from build123d import *

# Parameters (mm, degrees)
F0_R           = 25.1
F1_DEPTH       = 30
F2_R           = 2
F5_D           = 20
F5_DEPTH       = 190
F5_CSINK_D     = 22
F5_CSINK_ANGLE = 90
F5_TIP         = 6.0086061903


# Not quite as in the source:
# - a feature of the source that left no trace in its solid (it failed there, or was rolled back) is left out


with BuildPart() as f1:
    # F0 (on Front) → F1 (new body)
    with BuildSketch(Plane.XZ):
        with Locations((20.5169470484, 0)):
            Circle(F0_R)
    extrude(amount=F1_DEPTH)

    # F2
    f2_edges = [f1.edges().sort_by_distance(p)[0] for p in [
        (-4.583053, 0, 0),
    ]]
    fillet(f2_edges, radius=F2_R)

    # F5
    with Locations(Plane(origin=(0, 0, 0), x_dir=(-1, 0, 0), z_dir=(0, 1, 0))):
        with Locations((-20.5169470484, 0)):
            CounterSinkHole(F5_D / 2, F5_CSINK_D / 2, depth=F5_DEPTH, counter_sink_angle=F5_CSINK_ANGLE)
            with Locations((0, 0, -(F5_DEPTH + F5_TIP / 2))):  # 118° drill point
                Cone(0, F5_D / 2, F5_TIP, mode=Mode.SUBTRACT)


solid = f1.part
Check sheet for the modelled part. Datum: model origin and axes. Units: mm. Give positions to 0.01 mm unless a question says otherwise; leave off trailing zeros. Write each loop counter-clockwise with the first axis right and the second up, starting at its lowest first coordinate (ties: lowest second). Pieces come first, ordered by that corner, then holes. Notation, with made-up numbers: M 51.5,-23 L 63.5,-23 A15 cw 63.5,-15 Z; hole C 82,-28 d3. An arc over 180 degrees is marked long. Use one line per item in the form item = value.
(1) Section check A-A on z = 0. Record the boundary of the cut face in (x, y), plus the area to 3 significant figures.
Answer block:
outline = M -4.58,-30 L 10.52,-30 L 10.52,-1 L 9.52,0 L -2.58,0 A2 ccw -4.58,-2 Z; M 30.52,-30 L 45.62,-30 L 45.62,-2 A2 ccw 43.62,0 L 31.52,0 L 30.52,-1 Z
area = 903 mm2
(2) Section check B-B on y = -4. Record the boundary of the cut face in (x, z).
Answer block:
outline = C 20.52,0 d50.2; hole C 20.52,0 d20
(3) Depth check by flat-ended pin: P1, Ø5, axis at y = -23.5, z = -8.5, coming from the -X side; P2, Ø4, axis at y = -15.5, z = -14.5, coming from the -X side; P3, Ø6, axis at x = 30, y = -12, coming from the +Z side; P4, Ø18, axis at x = 20.52, z = 0, coming from the -Y side. Enter the tip coordinate at first touch or a pass-through.
Answer block:
P1 = -3.86
P2 = -1.25
P3 = 24.25
P4 = through
(4) Draft check along X on faces 1 (the cylindrical face through (43.703, -15.804, -9.613)), 2 (the cylindrical face through (12.58, -15.7, -6.08)), 3 (the flat face through (15, 0, -10)). Enter one of: pulls with the +X half, pulls with the -X half, needs draft (parallel to the pull), parting line crosses it, or undercut.
Answer block:
face_1 = parting line crosses it
face_2 = undercut
face_3 = needs draft
(5) Material ranges on line 1 along X through (y, z) = (-12.25, 4); line 2 along Z through (x, y) = (15.5, -17); line 3 along X through (y, z) = (-23.5, -13), recorded low to high.
Answer block:
line_1 = -4.26 to 11.35, 29.68 to 45.3
line_2 = -24.59 to -8.65, 8.65 to 24.59
line_3 = -0.95 to 41.99
